Work out the finished part from the listing and answer in its coordinate system (mm). A direction names the side the tool comes from. Round coordinates to 2 decimals unless told otherwise and drop trailing zeros. Order: outer loops, then holes, each group sorted by start corner. A loop starts at its lowest first (then second) coordinate and runs counter-clockwise, first axis right, second up. Notation, with made-up numbers: (62, -1.75) - (105, -1.75) arc R14 ccw to (105, 25.25) - close; hole circle Ø8 at (53.5, 0.5). An arc over 180 degrees is marked (long way). Put each result on its own line as item: value.
```python
from build123d import *

# Parameters (mm, degrees)
SALIENTE_EXTRUIR1_START = -1.5
SALIENTE_EXTRUIR1_DEPTH = 3
CROQUIS4_W              = 23.371648172
CROQUIS4_H              = 47.52448784
CORTAR_EXTRUIR3_DEPTH   = 10
CROQUIS5_W              = 9.999999994
CROQUIS5_H              = 3
CROQUIS5_W_2            = 9.999999993
CORTAR_EXTRUIR4_DEPTH   = 10
CROQUIS6_R              = 1.5
CORTAR_EXTRUIR5_DEPTH   = 10
REDONDEO1_R             = 5


# Read off the part's stored shape, not the designer's step: Saliente-Extruir1
with BuildPart() as part:
    # Saliente-Extruir1 outline → Saliente-Extruir1 (new body)
    with BuildSketch(Plane.XY.offset(SALIENTE_EXTRUIR1_START)):
        with BuildLine():
            ThreePointArc((492.916449572, 98.009593947), (492.452410006, 99.442022929), (491.249851225, 100.348134338))
            ThreePointArc((491.249851225, 100.348134338), (487.916517891, 105.062179546), (491.249851225, 109.776224754))
            ThreePointArc((491.249851225, 109.776224754), (492.452037009, 110.681812922), (492.916439741, 112.113480025))
            Line((492.916439741, 112.113480025), (492.916413331, 149.999679341))
            Line((492.916413331, 149.999679341), (410.416517891, 149.999679341))
            Line((410.416517891, 149.999679341), (410.416517891, 112.133247358))
            ThreePointArc((410.416517891, 112.133247358), (410.875276439, 110.689871685), (412.083184558, 109.776224754))
            ThreePointArc((412.083184558, 109.776224754), (415.416517891, 105.062179546), (412.083184558, 100.348134338))
            ThreePointArc((412.083184558, 100.348134338), (410.875276439, 99.434487407), (410.416517891, 97.991111734))
            Line((410.416517891, 97.991111734), (410.416517891, 52.008362374))
            ThreePointArc((410.416517891, 52.008362374), (410.875276439, 50.564986701), (412.083184558, 49.65133977))
            ThreePointArc((412.083184558, 49.65133977), (415.416517891, 44.937294562), (412.083184558, 40.223249354))
            ThreePointArc((412.083184558, 40.223249354), (410.875276439, 39.309602423), (410.416517891, 37.86622675))
            Line((410.416517891, 37.86622675), (410.416517891, -0.000320659))
            Line((410.416517891, -0.000320659), (492.916517891, -0.000320659))
            Line((492.916517891, -0.000320659), (492.916491488, 37.877716604))
            ThreePointArc((492.916491488, 37.877716604), (492.45443711, 39.314289338), (491.249851225, 40.223249354))
            ThreePointArc((491.249851225, 40.223249354), (487.916517891, 44.937294562), (491.249851225, 49.65133977))
            ThreePointArc((491.249851225, 49.65133977), (492.453865854, 50.559496169), (492.916481647, 51.994900607))
            Line((492.916481647, 51.994900607), (492.916449572, 98.009593947))
        make_face()
    extrude(amount=SALIENTE_EXTRUIR1_DEPTH)

    # Croquis4 → Cortar-Extruir3 (cut)
    with BuildSketch(Plane.XY.offset(1.5)):
        with Locations((455.222459901, 75.336681949)):
            Rectangle(CROQUIS4_W, CROQUIS4_H)
    extrude(amount=-CORTAR_EXTRUIR3_DEPTH, mode=Mode.SUBTRACT)

    # Croquis5 → Cortar-Extruir4 (cut)
    with BuildSketch(Plane(origin=(0, 0, -1.5), x_dir=(-1, 0, 0), z_dir=(0, 0, -1))):
        with Locations((-420.416517885, 27.399679341)):
            Rectangle(CROQUIS5_W, CROQUIS5_H)
        with Locations((-480.50829052, 27.399679341)):
            Rectangle(CROQUIS5_W_2, CROQUIS5_H)
        with Locations((-480.50829052, 122.599679342)):
            Rectangle(CROQUIS5_W_2, CROQUIS5_H)
        with Locations((-420.416517885, 122.599679342)):
            Rectangle(CROQUIS5_W, CROQUIS5_H)
    extrude(amount=-CORTAR_EXTRUIR4_DEPTH, mode=Mode.SUBTRACT)

    # Croquis6 → Cortar-Extruir5 (cut)
    with BuildSketch(Plane.XY.offset(1.5)):
        with Locations((460.461664074, 27.503843939)):
            Circle(CROQUIS6_R)
        with Locations((440.404261852, 27.568711017)):
            Circle(CROQUIS6_R)
        with Locations((440.404261852, 122.435783537)):
            Circle(CROQUIS6_R)
        with Locations((460.461664074, 122.500650615)):
            Circle(CROQUIS6_R)
    extrude(amount=-CORTAR_EXTRUIR5_DEPTH, mode=Mode.SUBTRACT)

    # Redondeo1
    redondeo1_edges = [part.edges().sort_by_distance(p)[0] for p in [
        (466.908283987, 99.098925869, 0),
        (466.908283987, 51.574438029, 0),
        (443.536635815, 51.574438029, 0),
        (443.536635815, 99.098925869, 0),
    ]]
    fillet(redondeo1_edges, radius=REDONDEO1_R)


solid = part.part
```
1) A cutting plane is placed at A-A on y = 86. Write down the section's boundary in (x, z).
Findings below:
outline: (410.42, -1.5) - (443.54, -1.5) - (443.54, 1.5) - (410.42, 1.5) - close; (466.91, -1.5) - (492.92, -1.5) - (492.92, 1.5) - (466.91, 1.5) - close
2) For faces 1 (the cylindrical face through (445.04, 53, -0.02)), 2 (the flat face through (492.916, 131, 0)), determine the directions among +Z, -Z, +X, -X, +Y, -Y from which every point of the face is accessible in a straight line to the end or side of a thin tool.
Findings below:
face 1: +Z, -Z
face 2: +Z, -Z, +X, +Y, -Y
3) For a pull along Y with two mould halves and no side action, classify faces 3 (the flat face through (410.417, 19, 0)), 4 (the flat face through (451, 0, 0)), 5 (the flat face through (415.417, 27, 0)) as pulls with the +Y half, pulls with the -Y half, needs draft (parallel to the pull), parting line crosses it, or undercut.
Findings below:
face 3: needs draft
face 4: pulls with the -Y half
face 5: undercut
4) Straight lines are drawn through the part: L1, parallel to Y at x = 477, z = -0.8; L2, parallel to X at y = 77, z = -0.7; L3, parallel to Y at x = 458.5, z = 1.3. For each, find the intervals that lie inside material, in ascending order. Write a range as from..to.
Findings below:
L1: y = 0..25.9, 28.9..121.1, 124.1..150
L2: x = 410.42..443.54, 466.91..492.92
L3: y = 0..51.57, 99.1..150
5) A cutting plane is placed at B-B on x = 452.5. Write down the section's boundary in (y, z), then the cut area to 3 significant figures.
Findings below:
outline: (0, -1.5) - (51.57, -1.5) - (51.57, 1.5) - (0, 1.5) - close; (99.1, -1.5) - (150, -1.5) - (150, 1.5) - (99.1, 1.5) - close
area: 307 mm2
6) A cutting plane is placed at C-C on z = -0.9. Give the number of separate pieces and of enclosed holes in the cut face, then the cut area to 3 significant figures.
Findings below:
separate pieces: 1
enclosed holes: 9
area: 11,000 mm2
7) Given pin 1 Ø2.5 at (x, y) = (460.46, 122.5) entering from +Z, flat-ended and moving along its own axis, determine where the tip first touches the part or whether it passes through.
Findings below:
pin 1: passes through
